Model file for the job. Use its own axes, mm. Face numbers are marked on the shaded views. A direction names the side the tool comes from. Round coordinates to 2 decimals unless told otherwise and drop trailing zeros. Use a Markdown table: item, result. Add a question column.
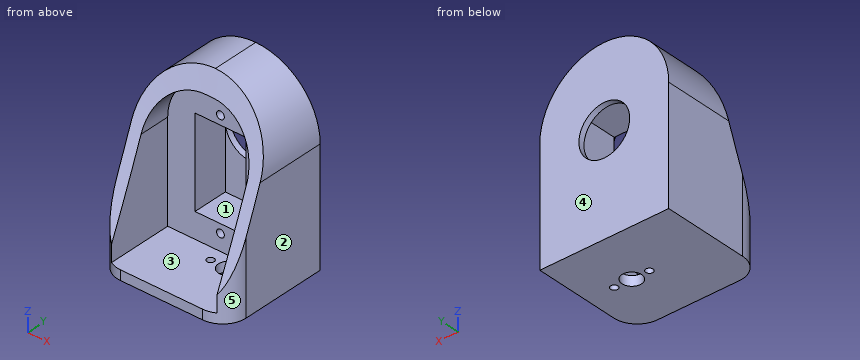
```python
from build123d import *

# Parameters (mm, degrees)
SKETCH1_W           = 33
SKETCH1_H           = 28
BOSS_EXTRUDE1_DEPTH = 46
CUT_EXTRUDE1_DEPTH  = 59.318093247
CUT_EXTRUDE4_START  = -3
CUT_EXTRUDE4_DEPTH  = 27
FILLET1_R           = 12.5
FILLET2_R           = 16.5
FILLET3_R           = 6
SKETCH5_W           = 13
SKETCH5_H           = 23
CUT_EXTRUDE8_DEPTH  = 9
SKETCH6_R           = 6.5
CUT_EXTRUDE9_DEPTH  = 56.592265809
SKETCH7_R           = 1
CUT_EXTRUDE10_DEPTH = 8
SKETCH8_R           = 0.925072744
SKETCH8_R_2         = 2.5
CUT_EXTRUDE11_DEPTH = 2.5


with BuildPart() as part:
    # Sketch1 → Boss-Extrude1 (new body)
    with BuildSketch(Plane.XY):
        Rectangle(SKETCH1_W, SKETCH1_H)
    extrude(amount=BOSS_EXTRUDE1_DEPTH)

    # Sketch3 → Cut-Extrude1 (cut, through all)
    with BuildSketch(Plane(origin=(16.5, 0, 0), x_dir=(0, 0, -1), z_dir=(1, 0, 0))):
        with BuildLine():
            Line((-46, 2), (-46, -14))
            Line((-46, -14), (-5, -14))
            add(Edge.make_bspline(
                [(-5, -14), (-25.11965555, -4.947029267), (-46, 2)],
                knots=[0, 0, 0, 1, 1, 1], degree=2))
        make_face()
    extrude(amount=-CUT_EXTRUDE1_DEPTH, mode=Mode.SUBTRACT)

    # Sketch4 → Cut-Extrude4 (cut)
    with BuildSketch(Plane(origin=(16.5, 0, 0), x_dir=(0, 0, -1), z_dir=(1, 0, 0)).offset(CUT_EXTRUDE4_START)):
        with BuildLine():
            Line((-5, -14), (-2.5, -14))
            Line((-2.5, -14), (-2.5, 3.5))
            Line((-2.5, 3.5), (-40.5, 3.5))
            Line((-40.5, 3.5), (-40.5, 0.128997137))
            add(Edge.make_bspline(
                [(-5, -14), (-22.463452761, -6.142205101), (-40.5, 0.128997137)],
                knots=[0, 0, 0, 1, 1, 1], degree=2))
        make_face()
    extrude(amount=-CUT_EXTRUDE4_DEPTH, mode=Mode.SUBTRACT)

    # Fillet1
    fillet1_edges = [part.edges().sort_by_distance(p)[0] for p in [
        (13.5, 1.814498569, 40.5),
        (-13.5, 1.814498569, 40.5),
    ]]
    fillet(fillet1_edges, radius=FILLET1_R)

    # Fillet2
    fillet2_edges = [part.edges().sort_by_distance(p)[0] for p in [
        (-16.5, 8, 46),
        (16.5, 8, 46),
    ]]
    fillet(fillet2_edges, radius=FILLET2_R - 0.0001)  # a hair under: the kernel refuses the full size

    # Fillet3
    fillet3_edges = [part.edges().sort_by_distance(p)[0] for p in [
        (-16.5, -14, 2.5),
        (16.5, -14, 2.5),
    ]]
    fillet(fillet3_edges, radius=FILLET3_R)

    # Sketch5 → Cut-Extrude8 (cut)
    with BuildSketch(Plane.XZ.offset(-3.5)):
        with Locations((0, 20.5)):
            Rectangle(SKETCH5_W, SKETCH5_H)
    extrude(amount=-CUT_EXTRUDE8_DEPTH, mode=Mode.SUBTRACT)

    # Sketch6 → Cut-Extrude9 (cut, through all)
    with BuildSketch(Plane.XZ.offset(-12.5)):
        with Locations(Location((0, 25.5, 0), (0, 0, 270))):
            Circle(SKETCH6_R)
    extrude(amount=-CUT_EXTRUDE9_DEPTH, mode=Mode.SUBTRACT)

    # Sketch7 → Cut-Extrude10 (cut)
    with BuildSketch(Plane.XZ.offset(-3.5)):
        with Locations(Location((0, 34.3, 0), (0, 0, 270))):
            Circle(SKETCH7_R)
        with Locations(Location((0, 6.7, 0), (0, 0, 270))):
            Circle(SKETCH7_R)
    extrude(amount=-CUT_EXTRUDE10_DEPTH, mode=Mode.SUBTRACT)

    # Sketch8 → Cut-Extrude11 (cut)
    with BuildSketch(Plane(origin=(0, 0, 0), x_dir=(-1, 0, 0), z_dir=(0, 0, -1))):
        with Locations((-9.5, 0)):
            Circle(SKETCH8_R)
        with Locations((-5, 0)):
            Circle(SKETCH8_R_2)
        with Locations((-0.5, 0)):
            Circle(SKETCH8_R)
    extrude(amount=-CUT_EXTRUDE11_DEPTH, mode=Mode.SUBTRACT)


solid = part.part
```
1) Pin check, flat tips, straight feed: pin 1 Ø5 at (y, z) = (1, 41) entering from -X; pin 2 Ø1.9 at (x, z) = (4.5, 28.5) entering from -Y; pin 3 Ø4 at (y, z) = (4.5, 38) entering from -X; pin 4 Ø14.5 at (x, z) = (1, 20) entering from -Y. Stop position of each tip, or through.
2) Tool access for the marked faces 1 and 2: list every direction of +Z, -Z, +X, -X, +Y, -Y with a clear straight run to the whole face (end or side of a thin tool).
3) Cut at A-A on x = 5. Count the separate pieces of the cut face and the enclosed holes in it, and give its area (3 significant figures).
4) Pull direction X, two halves, no side cores. Call the marked faces 3, 4 and 5: +X half, -X half, draft (parallel to the pull), parting line (faces both ways), or undercut.
5) Wall check: probe 1 along X at (y, z) = (-6.25, 14); probe 2 along X at (y, z) = (6, 6.7); probe 3 along Y at (x, z) = (5, 1). Give the ranges that are in metal, low to high. Write a range as from..to.
Established:
| question | item | result |
|---|---|---|
| 1 | pin 1 | stops at x = -13.83 |
| 1 | pin 2 | passes through |
| 1 | pin 3 | stops at x = -15.17 |
| 1 | pin 4 | stops at y = 3.5 |
| 2 | face 1 | -Y |
| 2 | face 2 | +Z, -Z, +X, +Y, -Y |
| 3 | separate pieces | 3 |
| 3 | enclosed holes | 0 |
| 3 | area | 301 mm^2 |
| 4 | face 3 | undercut |
| 4 | face 4 | draft |
| 4 | face 5 | +X half |
| 5 | probe 1 | x = -16.5..-13.5, 13.5..16.5 |
| 5 | probe 2 | x = -16.5..-1, 1..16.5 |
| 5 | probe 3 | y = -14..-2.5, 2.5..14 |
